Can you work these out from the model? Positions are in its coordinate system, mm. A direction names the side the tool comes from. Coordinates: 2 decimals unless noted, no trailing zeros. Order: outer loops, then holes, each group sorted by start corner. A loop starts at its lowest first (then second) coordinate and runs counter-clockwise, first axis right, second up. Notation, with made-up numbers: (-14, 12) -> (-7, 12) arc R34 cw to (-7, 44) -> close; hole circle Ø1 at (87, 67). An arc over 180 degrees is marked (long way). Answer as a JSON object with one key per item and string values. Group by question number.
(1) I want a section at A-A, the plane z = -31. List the corners of the cut face in (x, y) for me.
(2) I need wall thicknesses on line 1 (X direction, y = 5.5, z = -32); line 2 (Z direction, x = 14, y = 2); line 3 (X direction, y = 8.25, z = -19.5). Which ranges of each line are inside material? Lowest first, please.
(3) I want a section at D-D, the plane z = -19.5. List the corners of the cut face in (x, y) for me, plus the area to 3 significant figures.
(4) I want a section at B-B, the plane y = 13.75. List the corners of the cut face in (x, z) for me.
(5) For pin 1 (7.5 mm diameter, centred on x = -14, y = 6, fed in from -Z); pin 2 (3 mm diameter, centred on x = -9, z = -25.5, fed in from -Y); pin 3 (1 mm diameter, centred on x = -2, y = 10, fed in from -Z), each with a flat end and sliding along its axis, tell me the tip position at first contact or that it passes through.
(6) I want a section at C-C, the plane x = 0. List the corners of the cut face in (y, z) for me, plus the area to 3 significant figures.
(7) Which directions (+Z, -Z, +X, -X, +Y, -Y) give clear straight access to the entire face, cutting with the end or side of a thin tool? Please do faces 1 (the flat face through (19.627, 7, -30)), 2 (the flat face through (-30.422, 7, -18)).
(8) If we mould it in two halves opening along X, with no side actions, what happens to faces 3 (the flat face through (-25, 7, -35.207)), 4 (the flat face through (30.422, 7, -17)), 5 (the flat face through (-19.627, 7, -30)), 6 (the flat face through (-15, 7, -24.412))? For each: pulls with the +X half, pulls with the -X half, needs draft (parallel to the pull), parting line crosses it, or undercut.
from build123d import *

# Parameters (mm, degrees)
BOSS_EXTRUDE1_DEPTH = 15


with BuildPart() as part:
    # Sketch4 → Boss-Extrude1 (new body)
    with BuildSketch(Plane(origin=(0, 0, 0), x_dir=(1, 0, 0), z_dir=(0, 1, 0))):
        with BuildLine():
            Line((-30.42245721, 0), (30.42245721, 0))
            Line((30.42245721, 0), (30.42245721, 35.206633949))
            Line((30.42245721, 35.206633949), (19.627391749, 35.206633949))
            Line((19.627391749, 35.206633949), (19.627391749, 24.411568487))
            Line((19.627391749, 24.411568487), (10.446516771, 24.411568487))
            ThreePointArc((10.446516771, 24.411568487), (0, 13.965051717), (-10.446516771, 24.411568487))
            Line((-10.446516771, 24.411568487), (-19.627391749, 24.411568487))
            Line((-19.627391749, 24.411568487), (-19.627391749, 35.206633949))
            Line((-19.627391749, 35.206633949), (-30.42245721, 35.206633949))
            Line((-30.42245721, 35.206633949), (-30.42245721, 0))
        make_face()
    extrude(amount=BOSS_EXTRUDE1_DEPTH)


solid = part.part
Computed values:
{
 "1": {"outline": "(-30.42, 0) -> (-19.63, 0) -> (-19.63, 15) -> (-30.42, 15) -> close; (19.63, 0) -> (30.42, 0) -> (30.42, 15) -> (19.63, 15) -> close"},
 "2": {"line 1": "x = -30.42 to -19.63, 19.63 to 30.42", "line 2": "z = -24.41 to 0", "line 3": "x = -30.42 to -9.22, 9.22 to 30.42"},
 "3": {"outline": "(-30.42, 0) -> (-9.22, 0) -> (-9.22, 15) -> (-30.42, 15) -> close; (9.22, 0) -> (30.42, 0) -> (30.42, 15) -> (9.22, 15) -> close", "area": "636 mm2"},
 "4": {"outline": "(-30.42, -35.21) -> (-19.63, -35.21) -> (-19.63, -24.41) -> (-10.45, -24.41) arc R10.45 cw to (10.45, -24.41) -> (19.63, -24.41) -> (19.63, -35.21) -> (30.42, -35.21) -> (30.42, 0) -> (-30.42, 0) -> close"},
 "5": {"pin 1": "stops at z = -24.41", "pin 2": "passes through", "pin 3": "stops at z = -14.27"},
 "6": {"outline": "(0, -13.97) -> (15, -13.97) -> (15, 0) -> (0, 0) -> close", "area": "209 mm2"},
 "7": {"face 1": "-Z, +Y, -Y", "face 2": "+Z, -Z, -X, +Y, -Y"},
 "8": {"face 3": "needs draft", "face 4": "pulls with the +X half", "face 5": "undercut", "face 6": "undercut"}
}
